Here's how the part is built. I have some questions about the finished solid (model axes, mm). A direction names the side the tool comes from. Coordinates: 2 decimals unless noted, no trailing zeros. Write each loop counter-clockwise with the first axis right and the second up, starting at its lowest first coordinate (ties: lowest second). Pieces come first, ordered by that corner, then holes. Notation, with made-up numbers: M 82,25.25 L 132,25.25 A30 ccw 132,58.25 Z; hole C 13.5,-2.75 d11. An arc over 180 degrees is marked long. Use one line per item in the form item = value. Start each with the question number.
1. Thinking about a two-plate mould opening in Z: for faces 1 (the face through (-1, 6, -37.5)), 2 (the face through (1, 0, 1)), 3 (the face through (0, 7, -35)), which applies, released by +Z, released by -Z, zero draft, split by the parting line, or undercut?
2. Please list where these lines run through material, in increasing order: line 1 along X through (y, z) = (6, -14.5); line 2 along Y through (x, z) = (-11, -22). Write a range as [from, to].
3. I'm going to push a flat-ended pin straight in: pin 1 Ø21 at (x, z) = (9, 12.5) entering from +Y. Where does the tip first touch, or does it pass through?
4. I want a section at C-C, the plane x = -22.5. List the corners of the cut face in (y, z) for me.
5. I want a section at A-A, the plane y = 6.75. List the corners of the cut face in (x, z) for me, plus the area to 3 significant figures.
6. On a 3-axis mill with a long thin cutter (end or side, diameter ignored), from which of +Z, -Z, +X, -X, +Y, -Y can I reach the whole of each face in a straight line? I mean faces 4 (the face through (-35, 7, 0)), 5 (the face through (1, 6, 37.5)). Say none if no direction works.
7. I want a section at B-B, the plane z = 6.5. List the corners of the cut face in (x, y) for me, plus the area to 3 significant figures.
Autodesk Inventor part; units mm, degrees
ref_plane "YZ Plane" through (0, 0, 0) normal (1, 0, 0) x (0, 1, 0)
ref_plane "XZ Plane" through (0, 0, 0) normal (0, 1, 0) x (-1, 0, 0)
ref_plane "XY Plane" through (0, 0, 0) normal (0, 0, 1) x (1, 0, 0)
sketch "Sketch1" plane through (0, 0, 0) normal (0, 1, 0) x (-1, 0, 0)
  line L0 (-37.5, 37.5) -> (37.5, 37.5)
  line L1 (37.5, 37.5) -> (37.5, -37.5)
  line L2 (37.5, -37.5) -> (-37.5, -37.5)
  line L3 (-37.5, -37.5) -> (-37.5, 37.5)
  line L4 (-37.5, 37.5) -> (37.5, -37.5) construction
  line L5 (37.5, 37.5) -> (-37.5, -37.5) construction
  line L6 (-35, -35) -> (35, -35)
  line L7 (35, -35) -> (35, 35)
  line L8 (35, 35) -> (-35, 35)
  line L9 (-35, 35) -> (-35, -35)
  line L10 (-35, -35) -> (35, 35) construction
  line L11 (35, -35) -> (-35, 35) construction
  point P0 (0, 0)
  dimension "d0" = 75
  dimension "d1" = 75
  dimension "d2" = 70
  dimension "d3" = 70
extrude "Extrusion1" add sketch "Sketch1" along normal blind 12
extrude "Extrusion2" add sketch "Sketch1" along normal blind 2.5 contours L9 L8 L7 L6
properties part number "boxCap"
Answer list:
q1.face_1 = released by -Z
q1.face_2 = zero draft
q1.face_3 = undercut
q2.line_1 = [-37.5, -35], [35, 37.5]
q2.line_2 = [0, 2.5]
q3.pin_1 = 2.5
q4.outline = M 0,-37.5 L 12,-37.5 L 12,-35 L 2.5,-35 L 2.5,35 L 12,35 L 12,37.5 L 0,37.5 Z
q5.outline = M -37.5,-37.5 L 37.5,-37.5 L 37.5,37.5 L -37.5,37.5 Z; hole M -35,-35 L 35,-35 L 35,35 L -35,35 Z
q5.area = 725 mm²
q6.face_4 = +Y
q6.face_5 = +Z, +X, -X, +Y, -Y
q7.outline = M -37.5,0 L 37.5,0 L 37.5,12 L 35,12 L 35,2.5 L -35,2.5 L -35,12 L -37.5,12 Z
q7.area = 235 mm²
